Geometry: final body of the model. Coordinates: model frame, mm. Face numbers are marked on the shaded views. A direction names the side the tool comes from. Give positions to 0.01 mm unless a question says otherwise; leave off trailing zeros. Write each loop counter-clockwise with the first axis right and the second up, starting at its lowest first coordinate (ties: lowest second). Pieces come first, ordered by that corner, then holes. Notation, with made-up numbers: (70, -7) -> (99, -7) arc R18 cw to (99, 3) -> close; hole circle Ø2 at (79.5, 72.5). An arc over 180 degrees is marked (long way). Answer as a JSON object with one key per item and string values. Group by question number.
(1) Section query B-B on y = 2.5. Output: boundary loops of the cut face in (x, z), plus the area to 3 significant figures.
(2) Section query C-C on z = 3.25. Output: boundary loops of the cut face in (x, y).
(3) Section query D-D on y = 11. Output: boundary loops of the cut face in (x, z).
(4) Draft query along Y for the marked faces 1, 2 and 3. Return one class per face: +Y half, -Y half, draft (parallel to the pull), parting line (faces both ways), or undercut.
(5) Material intervals for probe 1 along Y at (x, z) = (2.5, -0.75); probe 2 along Z at (x, y) = (0, 5.25); probe 3 along Z at (x, y) = (0, 9), sorted ascending.
(6) Contact query for flat-ended pins moving along their axis: pin 1 Ø1 at (x, z) = (0.5, 1.5) entering from -Y; pin 2 Ø3 at (x, z) = (2, -2) entering from -Y; pin 3 Ø3 at (y, z) = (5.5, 1.5) entering from +X. Output: stop coordinate, or through.
(7) Set-up query: the marked faces 4, 5, 6 and 7. Return all of +Z, -Z, +X, -X, +Y, -Y with unobstructed straight access to the full face (end or side cutting, diameter ignored); none if empty.
Autodesk Inventor part; units mm, degrees
ref_plane "YZ Plane" through (0, 0, 0) normal (1, 0, 0) x (0, 1, 0)
ref_plane "XZ Plane" through (0, 0, 0) normal (0, 1, 0) x (-1, 0, 0)
ref_plane "XY Plane" through (0, 0, 0) normal (0, 0, 1) x (1, 0, 0)
sketch "Эскиз1" plane through (0, 0, 0) normal (0, 0, 1) x (1, 0, 0)
  line L0 (0, 0) -> (0, 15)
  line L1 (0, 12.5) -> (3, 12.5)
  line L2 (2.4004, 2) -> (4.0415, 2)
  line L3 (2.5, 5) -> (4.0415, 5)
  line L4 (2.5, 6.5) -> (3, 6.5)
  line L5 (0, 0) -> (1, 0)
  line L6 (2.5, 6.5) -> (2.5, 5)
  line L7 (3, 12.5) -> (3, 6.5)
  line L8 (1, 0) -> (2.4004, 2)
  line L9 (4.0415, 5) -> (4.0415, 2)
  line L10 (0, 12.5) -> (0, 0)
  dimension "d0" = 15
  dimension "d1" = 12.5
  dimension "d2" = 10.5
  dimension "d3" = 7.5
  dimension "d4" = 6
  dimension "d6" = 5
  dimension "d7" = 6
  dimension "d8" = 125
  dimension "d11" = 8.083
  dimension "d44" = 2
revolve "Вращение1" add sketch "Эскиз1" angle 360 about axis through (0, 0, 0) along (0, 1, 0)
chamfer "Фаска1" distance 0.25 angle 45 2 edges at (-3, 12.5, 0) (-3, 6.5, 0)
thread "Резьба1"
sketch "Эскиз2" plane through (0, 12.5, 0) normal (0, 1, 0) x (1, 0, 0)
  point P0 (0, 0)
  point P1 (0, 0)
sketch "Эскиз3" plane through (0, 0, 0) normal (0, -1, 0) x (1, 0, 0)
  point P0 (0, 0)
  point P1 (0, 0)
hole "Отверстие2" at (0, 12.5, 0) direction (0, -1, 0) diameter 2 depth 10.9 tip angle 130
chamfer "Фаска2" distance 0.2 angle 45 1 edges at (0, 12.5, -1)
hole "Отверстие3" at (0, 0, 0) direction (0, 1, 0) diameter 0.8 depth 1.6
sketch "Эскиз4" plane through (0, 2, 0) normal (0, -1, 0) x (1, 0, 0)
  circle A0 centre (0, 0) radius 0.4
  circle A1 centre (0, 0) radius 4.0415
  line L0 (4.0415, 0) -> (2.0208, -3.5)
  line L1 (2.0208, -3.5) -> (-2.0207, -3.5)
  line L2 (-2.0207, -3.5) -> (-4.0415, 0)
  line L3 (-4.0415, 0) -> (-2.0208, 3.5)
  line L4 (-2.0208, 3.5) -> (2.0207, 3.5)
  line L5 (2.0207, 3.5) -> (4.0415, 0)
extrude "Выдавливание1" cut sketch "Эскиз4" against normal blind 3 contours L5 A1 | A1 L0 | L4 A1 | A1 L1 | L3 A1 | A1 L2
properties part number "nozzle-0,8"
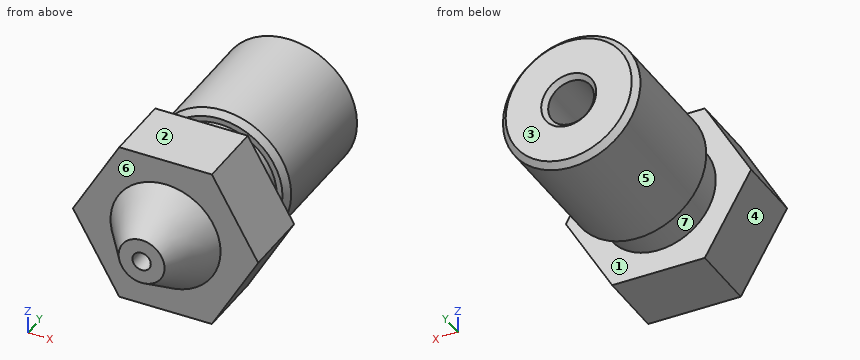
Answer list:
{
 "1": {"outline": "(-4.04, 0) -> (-2.02, -3.5) -> (2.02, -3.5) -> (4.04, 0) -> (2.02, 3.5) -> (-2.02, 3.5) -> close; hole circle Ø2 at (0, 0)", "area": "39.3 mm2"},
 "2": {"outline": "(-2.17, 2) -> (2.17, 2) -> (2.17, 5) -> (-2.17, 5) -> close"},
 "3": {"outline": "circle Ø6 at (0, 0); hole circle Ø2 at (0, 0)"},
 "4": {"face 1": "undercut", "face 2": "draft", "face 3": "+Y half"},
 "5": {"probe 1": "2 to 5, 6.5 to 12.5", "probe 2": "-2.5 to -1, 1 to 2.5", "probe 3": "-3 to -1, 1 to 3"},
 "6": {"pin 1": "y = 0.12", "pin 2": "y = 0.47", "pin 3": "x = 3.99"},
 "7": {"face 4": "-Z, -X, +Y, -Y", "face 5": "+Y", "face 6": "-Y", "face 7": "none"}
}
